The drawing under review shows one solid part. Ordinate dimensions are in mm from its lowest x, y, z. Coordinates: 2 decimals unless noted, no trailing zeros. Write each loop counter-clockwise with the first axis right and the second up, starting at its lowest first coordinate (ties: lowest second). Pieces come first, ordered by that corner, then holes. Notation, with made-up numbers: M 3.25,-30.5 L 52.25,-30.5 A17 ccw 52.25,1.5 Z; hole C 25,72.25 d1. An arc over 180 degrees is marked long. Write item = value, one per line.
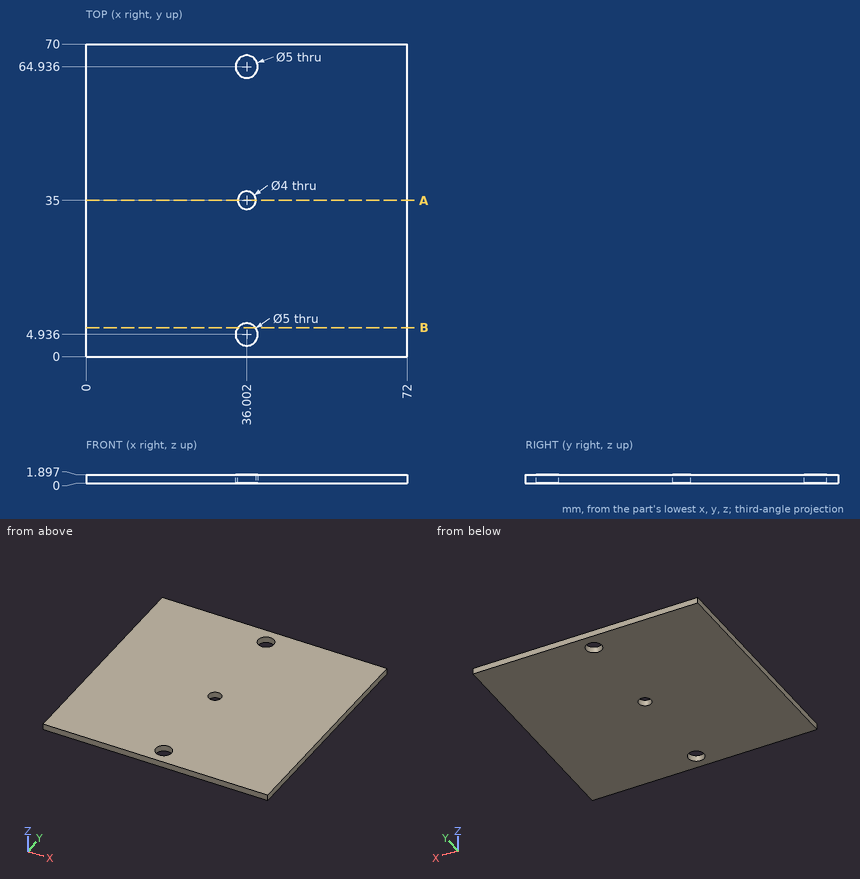
Q1. Consider section A-A, the plane y = 35. State the section outline as (x, z) points, and give its area (3 significant figures).
Check result:
outline = M 0,0 L 34,0 L 34,1.9 L 0,1.9 Z; M 38,0 L 72,0 L 72,1.9 L 38,1.9 Z
area = 129 mm²
Q2. Wall thickness on line 1 (Y direction, x = 36, z = 1.7) (1 decimal); line 2 (Y direction, x = 37.5, z = 1.4) (1 decimal); line 3 (X direction, y = 5.5, z = 1.55): over which ranges is each line inside the solid? List them lowest first.
Check result:
line_1 = 0 to 2.4, 7.4 to 33, 37 to 62.4, 67.4 to 70
line_2 = 0 to 2.9, 6.9 to 33.7, 36.3 to 62.9, 66.9 to 70
line_3 = 0 to 33.57, 38.44 to 72
Q3. Consider section B-B, the plane y = 6.5. State the section outline as (x, z) points, and give its area (3 significant figures).
Check result:
outline = M 0,0 L 34.05,0 L 34.05,1.9 L 0,1.9 Z; M 37.95,0 L 72,0 L 72,1.9 L 37.95,1.9 Z
area = 129 mm²
